from build123d import *

# Parameters (mm, degrees)
SKETCH1_W           = 35
SKETCH1_H           = 140
SKETCH1_R           = 3
BOSS_EXTRUDE1_DEPTH = 4
SKETCH2_W           = 35
SKETCH2_H           = 8
BOSS_EXTRUDE2_DEPTH = 4


with BuildPart() as part:
    # Sketch1 → Boss-Extrude1 (new body)
    with BuildSketch(Plane.XY):
        Rectangle(SKETCH1_W, SKETCH1_H)
        with Locations((0.277177956, -45.903341346)):
            Circle(SKETCH1_R, mode=Mode.SUBTRACT)
    extrude(amount=BOSS_EXTRUDE1_DEPTH)

    # Sketch2 → Boss-Extrude2 (add)
    with BuildSketch(Plane(origin=(0, 70, 0), x_dir=(1, 0, 0), z_dir=(0, 1, 0))):
        with Locations((0, -2)):
            Rectangle(SKETCH2_W, SKETCH2_H)
    extrude(amount=-BOSS_EXTRUDE2_DEPTH)


solid = part.part
For this review, take the finished solid that the model builds, in its own axes (mm). A direction names the side the tool comes from. Round coordinates to 2 decimals unless told otherwise and drop trailing zeros. Write each loop counter-clockwise with the first axis right and the second up, starting at its lowest first coordinate (ties: lowest second). Pieces come first, ordered by that corner, then holes. Notation, with made-up numbers: (17, 50.5) - (40, 50.5) arc R13 cw to (40, 66.5) - close; hole circle Ø11 at (10, 38.5). An arc over 180 degrees is marked (long way). Write item = value, one per line. Start each with the question number.
1. Draft analysis for pull direction X (two halves, no side actions). For faces 1 (the face through (0, 70, 2)), 2 (the face through (17.5, 1, 2)), 3 (the face through (1.89, -43.374, 1.972)), state which applies: released by +X, released by -X, zero draft, split by the parting line, or undercut.
2. Wall thickness on L1, parallel to Z at x = 10.5, y = -2; L2, parallel to Y at x = -11, z = -0.5; L3, parallel to Y at x = -2, z = 3.25: over which ranges is each line inside the solid? List them lowest first.
3. Consider section B-B on y = 35. State the section outline as (x, z) points.
4. Consider section A-A on x = 12. State the section outline as (y, z) points.
5. For pin 1 Ø4 at (x, y) = (11.5, -51.5) entering from +Z; pin 2 Ø3 at (x, y) = (-10.5, 3) entering from -Z; pin 3 Ø5.5 at (x, y) = (0.28, -45.9) entering from +Z, all flat-tipped, find the tip position at first contact; note any pin that passes through.
6. For faces 4 (the face through (0, 68, -2)), 5 (the face through (0, -1, 4)), 6 (the face through (0, -1, 0)), list the 3-axis set-ups (+Z, -Z, +X, -X, +Y, -Y) from which the entire face can be reached by the end or side of a thin tool; tool diameter is ignored.
Evaluation:
q1.face_1 = zero draft
q1.face_2 = released by +X
q1.face_3 = undercut
q2.L1 = 0 to 4
q2.L2 = 66 to 70
q2.L3 = -70 to -47.86, -43.95 to 70
q3.outline = (-17.5, 0) - (17.5, 0) - (17.5, 4) - (-17.5, 4) - close
q4.outline = (-70, 0) - (66, 0) - (66, -2) - (70, -2) - (70, 6) - (66, 6) - (66, 4) - (-70, 4) - close
q5.pin_1 = 4
q5.pin_2 = 0
q5.pin_3 = through
q6.face_4 = -Z, +X, -X, +Y, -Y
q6.face_5 = +Z, +X, -X, -Y
q6.face_6 = -Z, +X, -X, -Y
